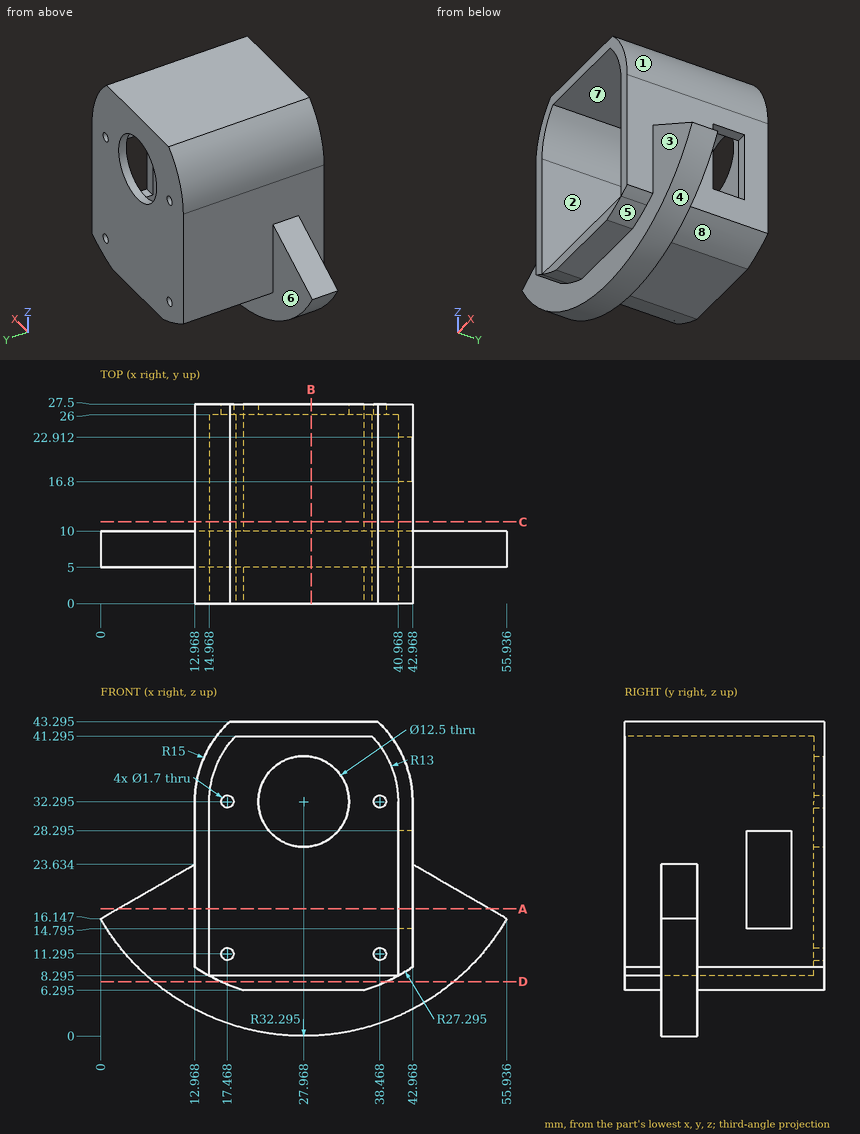
Here's the drawing with two shaded views (mm, measured from the low corner). I have some questions. A direction names the side the tool comes from. Give positions to 0.01 mm unless a question says otherwise; leave off trailing zeros. Order: outer loops, then holes, each group sorted by start corner. A loop starts at its lowest first (then second) coordinate and runs counter-clockwise, first axis right, second up. Notation, with made-up numbers: M -2.75,61 L 24.25,61 A15 cw 24.25,89 Z; hole C 54,14.25 d6. An arc over 180 degrees is marked long. Answer as a JSON object with one key per item and string values. Group by question number.
1) Suppose I cut it at B-B, the plane x = 29. Write out the boundary of the cut face in (y, z) (1 decimal).
2) Suppose I cut it at A-A, the plane z = 17.5. Write out the boundary of the cut face in (x, y).
3) Suppose I cut it at C-C, the plane y = 11.25. Write out the boundary of the cut face in (x, z) (1 decimal), plus the area to 3 significant figures.
4) On a 3-axis mill with a long thin cutter (end or side, diameter ignored), from which of +Z, -Z, +X, -X, +Y, -Y can I reach the whole of each face in a straight line? I mean the marked faces 5, 6, 7 and 8. Say none if no direction works.
5) Suppose I cut it at D-D, the plane z = 7.5. Write out the boundary of the cut face in (x, y) (1 decimal).
6) Please list where these lines run through material, in increasing order: L1, parallel to Z at x = 28, y = 6 (1 decimal); L2, parallel to X at y = 1.5, z = 9.5; L3, parallel to Z at x = 27, y = 22.75 (1 decimal). Write a range as [from, to].
7) We'd pull the mould along Z, two halves only. Please class the marked faces 1, 2, 3 and 4: pulls with the +Z half, pulls with the -Z half, needs draft (parallel to the pull), parting line crosses it, or undercut.
8) I'm going to push flat-ended pins straight in: pin 1 Ø1.5 at (x, z) = (38.47, 11.29) entering from +Y; pin 2 Ø12 at (x, y) = (43, 18) entering from -Z; pin 3 Ø8 at (y, z) = (17, 24) entering from +X; pin 4 Ø2.5 at (x, z) = (17.47, 32.29) entering from -Y. Where does each tip first touch, or does it pass through?
Results found:
{
 "1": {"outline": "M 0,6.3 L 5,6.3 L 5,0 L 10,0 L 10,6.3 L 27.5,6.3 L 27.5,26.1 L 26,26.1 L 26,8.3 L 0,8.3 Z; M 0,41.3 L 26,41.3 L 26,38.5 L 27.5,38.5 L 27.5,43.3 L 0,43.3 Z"},
 "2": {"outline": "M 2.34,5 L 12.97,5 L 12.97,0 L 14.97,0 L 14.97,26 L 40.97,26 L 40.97,22.91 L 42.97,22.91 L 42.97,27.5 L 12.97,27.5 L 12.97,10 L 2.34,10 Z; M 40.97,0 L 42.97,0 L 42.97,5 L 53.59,5 L 53.59,10 L 42.97,10 L 42.97,16.8 L 40.97,16.8 Z"},
 "3": {"outline": "M 13,9.5 A27.3 ccw 19.7,6.3 L 36.3,6.3 A27.3 ccw 43,9.5 L 43,32.3 A15 ccw 38.2,43.3 L 17.8,43.3 A15 ccw 13,32.3 Z; hole M 15,8.3 L 41,8.3 L 41,32.3 A13 ccw 37.3,41.3 L 18.6,41.3 A13 ccw 15,32.3 Z", "area": "221 mm²"},
 "4": {"face 5": "-Z, +X, -Y", "face 6": "-Z, +Y", "face 7": "-Y", "face 8": "-Z, +X, +Y"},
 "5": {"outline": "M 7.3,5 L 16.6,5 L 16.6,0 L 39.4,0 L 39.4,5 L 48.7,5 L 48.7,10 L 39.4,10 L 39.4,27.5 L 16.6,27.5 L 16.6,10 L 7.3,10 Z"},
 "6": {"L1": "[0, 8.3], [41.3, 43.3]", "L2": "[12.97, 14.97], [40.97, 42.97]", "L3": "[6.3, 8.3], [41.3, 43.3]"},
 "7": {"face 1": "pulls with the +Z half", "face 2": "undercut", "face 3": "needs draft", "face 4": "pulls with the -Z half"},
 "8": {"pin 1": "through", "pin 2": "z = 6.54", "pin 3": "x = 42.97", "pin 4": "y = 26"}
}
